```python
from build123d import *

# Parameters (mm, degrees)
BOSS_EXTRUDE1_DEPTH  = 5
M3_CLEARANCE_HOLE1_D = 3.4
SKETCH2_R            = 14.75
BOSS_EXTRUDE2_DEPTH  = 4
SKETCH4_R            = 12
CUT_EXTRUDE1_DEPTH   = 3.5
CUT_EXTRUDE2_DEPTH   = 2.5
SKETCH8_R            = 3.75
CUT_EXTRUDE3_DEPTH   = 31.203476621
SKETCH3_R            = 1.7
CUT_EXTRUDE4_DEPTH   = 32.032241298


with BuildPart() as part:
    # Sketch1 → Boss-Extrude1 (new body)
    with BuildSketch(Plane(origin=(0, 0, 0), x_dir=(1, 0, 0), z_dir=(0, 1, 0))):
        Polygon((-21, 15), (-21, -15), (-15, -21), (15, -21), (21, -15), (21, 15), (15, 21), (-15, 21), align=None)
    extrude(amount=BOSS_EXTRUDE1_DEPTH)

    # M3 Clearance Hole1 (through all)
    with Locations(Plane(origin=(0, 5, 0), x_dir=(1, 0, 0), z_dir=(0, 1, 0))):
        with Locations((15.5, 15.5), (-15.5, 15.5), (-15.5, -15.5), (15.5, -15.5)):
            Hole(M3_CLEARANCE_HOLE1_D / 2)

    # Sketch2 → Boss-Extrude2 (add)
    with BuildSketch(Plane(origin=(0, 5, 0), x_dir=(1, 0, 0), z_dir=(0, 1, 0))):
        with Locations(Location((0, 0, 0), (0, 0, 270))):
            Circle(SKETCH2_R)
    extrude(amount=BOSS_EXTRUDE2_DEPTH)

    # Sketch4 → Cut-Extrude1 (cut)
    with BuildSketch(Plane(origin=(0, 0, 0), x_dir=(-1, 0, 0), z_dir=(0, -1, 0))):
        with Locations(Location((0, 0, 0), (0, 0, 90))):
            Circle(SKETCH4_R)
    extrude(amount=-CUT_EXTRUDE1_DEPTH, mode=Mode.SUBTRACT)

    # Sketch7 → Cut-Extrude2 (cut)
    with BuildSketch(Plane.XZ.offset(-3.5)):
        Polygon((3.645190528, 2.104551733), (6.495190528, 0.459103466), (9.345190528, 2.104551733), (9.345190528, 5.395448267), (6.495190528, 7.040896534), (3.645190528, 5.395448267), align=None)
        Polygon((0, 4.209103466), (2.85, 5.854551733), (2.85, 9.145448267), (0, 10.790896534), (-2.85, 9.145448267), (-2.85, 5.854551733), align=None)
        Polygon((3.645190528, -2.104551733), (3.645190528, -5.395448267), (6.495190528, -7.040896534), (9.345190528, -5.395448267), (9.345190528, -2.104551733), (6.495190528, -0.459103466), align=None)
        Polygon((0, -4.209103466), (-2.85, -5.854551733), (-2.85, -9.145448267), (0, -10.790896534), (2.85, -9.145448267), (2.85, -5.854551733), align=None)
        Polygon((-3.645190528, -2.104551733), (-6.495190528, -0.459103466), (-9.345190528, -2.104551733), (-9.345190528, -5.395448267), (-6.495190528, -7.040896534), (-3.645190528, -5.395448267), align=None)
        Polygon((-3.645190528, 2.104551733), (-3.645190528, 5.395448267), (-6.495190528, 7.040896534), (-9.345190528, 5.395448267), (-9.345190528, 2.104551733), (-6.495190528, 0.459103466), align=None)
    extrude(amount=-CUT_EXTRUDE2_DEPTH, mode=Mode.SUBTRACT)

    # Sketch8 → Cut-Extrude3 (cut, through all)
    with BuildSketch(Plane.XZ.offset(-3.5)):
        with Locations(Location((0, 0, 0), (0, 0, 270))):
            Circle(SKETCH8_R)
    extrude(amount=-CUT_EXTRUDE3_DEPTH, mode=Mode.SUBTRACT)

    # Sketch3 → Cut-Extrude4 (cut, through all)
    with BuildSketch(Plane(origin=(0, 9, 0), x_dir=(1, 0, 0), z_dir=(0, 1, 0))):
        with Locations(Location((0, 7.5, 0), (0, 0, 270))):
            Circle(SKETCH3_R)
        with Locations(Location((6.495690528, 3.750866025, 0), (0, 0, 270))):
            Circle(SKETCH3_R)
        with Locations(Location((6.496690528, -3.749133975, 0), (0, 0, 270))):
            Circle(SKETCH3_R)
        with Locations(Location((0.002, -7.5, 0), (0, 0, 270))):
            Circle(SKETCH3_R)
        with Locations(Location((-6.493690528, -3.750866025, 0), (0, 0, 270))):
            Circle(SKETCH3_R)
        with Locations(Location((-6.494690528, 3.749133975, 0), (0, 0, 270))):
            Circle(SKETCH3_R)
    extrude(amount=-CUT_EXTRUDE4_DEPTH, mode=Mode.SUBTRACT)


solid = part.part
```
Geometry: final body of the model. Coordinates: model frame, mm. A direction names the side the tool comes from. Round coordinates to 2 decimals unless told otherwise and drop trailing zeros. Loops run counter-clockwise (first coordinate to the right, second up) from the corner with the lowest first, then second, coordinate; pieces in that order, holes last.
Item 1: Contact query for flat-ended pins moving along their axis: P1, Ø12, axis at x = -4, z = -3.5, coming from the -Y side; P2, Ø4, axis at x = 15.5, z = 15.5, coming from the +Y side; P3, Ø3, axis at x = 0, z = -8.5, coming from the -Y side. Output: stop coordinate, or through.
Checked values:
P1: stops at y = 3.5
P2: stops at y = 5
P3: stops at y = 6
Item 2: Line query: L1, parallel to X at y = 1.8, z = 0; L2, parallel to Z at x = -16.5, y = 2; L3, parallel to X at y = 4.5, z = -9. Output: solid intervals per line, ascending.
Checked values:
L1: x = -21 to -12, 12 to 21
L2: z = -19.5 to -16.87, -14.13 to 14.13, 16.87 to 19.5
L3: x = -21 to -2.85, 2.85 to 21
Item 3: Section D-D, the plane y = 4. State how many separate pieces and enclosed holes the cut face has, plus the area to 3 significant figures.
Checked values:
separate pieces: 1
enclosed holes: 11
area: 1,440 mm2
Item 4: Section C-C, the plane y = 6.5. Output: boundary loops of the cut face in (x, z).
Checked values:
outline: circle Ø29.5 at (0, 0); hole circle Ø3.4 at (-6.49, -3.75); hole circle Ø3.4 at (-6.49, 3.75); hole circle Ø7.5 at (0, 0); hole circle Ø3.4 at (0, -7.5); hole circle Ø3.4 at (0, 7.5); hole circle Ø3.4 at (6.5, -3.75); hole circle Ø3.4 at (6.5, 3.75)
Item 5: Section B-B, the plane x = -15.5. Output: boundary loops of the cut face in (y, z), plus the area to 3 significant figures.
Checked values:
outline: (0, -20.5) - (5, -20.5) - (5, -17.2) - (0, -17.2) - close; (0, -13.8) - (5, -13.8) - (5, 13.8) - (0, 13.8) - close; (0, 17.2) - (5, 17.2) - (5, 20.5) - (0, 20.5) - close
area: 171 mm2
Item 6: Mould query, pull axis X, two halves, no side actions, for faces 1 (the flat face through (18, 2, -18)), 2 (the flat face through (-18, 2, -18)), 3 (the flat face through (-1.3, 6, 6.1)). Classes: released by +X, released by -X, zero draft, split by the parting line, or undercut.
Checked values:
face 1: released by +X
face 2: released by -X
face 3: undercut
Item 7: Section A-A, the plane z = -15.5. Output: boundary loops of the cut face in (x, y), plus the area to 3 significant figures.
Checked values:
outline: (-20.5, 0) - (-17.2, 0) - (-17.2, 5) - (-20.5, 5) - close; (-13.8, 0) - (13.8, 0) - (13.8, 5) - (-13.8, 5) - close; (17.2, 0) - (20.5, 0) - (20.5, 5) - (17.2, 5) - close
area: 171 mm2
Item 8: Reachability of faces 4 (the flat face through (-3.645, 5, -4)), 5 (the cylindrical face through (-1.03, 7.52, 6.15)) from +Z, -Z, +X, -X, +Y, -Y: full face, straight path, thin tool, end or side. Return the list, or none.
Checked values:
face 4: -Y
face 5: +Y, -Y
